```python
from build123d import *

# Parameters (mm, degrees)
SKETCH2_R           = 8.25
BOSS_EXTRUDE1_DEPTH = 5


with BuildPart() as part:
    # Sketch2 → Boss-Extrude1 (new, symmetric)
    with BuildSketch(Plane.XY.offset(-25)):
        Polygon((227.33813101, -85), (237.93813101, -85), (237.93813101, -64.7), (267.93813101, -64.7), (267.93813101, -144.7), (247.93813101, -164.7), (217.33813101, -164.7), (197.33813101, -144.7), (197.33813101, -64.7), (227.33813101, -64.7), align=None)
        with Locations(Location((232.63813101, -149.7, 0), (0, 0, 180))):
            Circle(SKETCH2_R, mode=Mode.SUBTRACT)
    extrude(amount=BOSS_EXTRUDE1_DEPTH, both=True)


solid = part.part
```
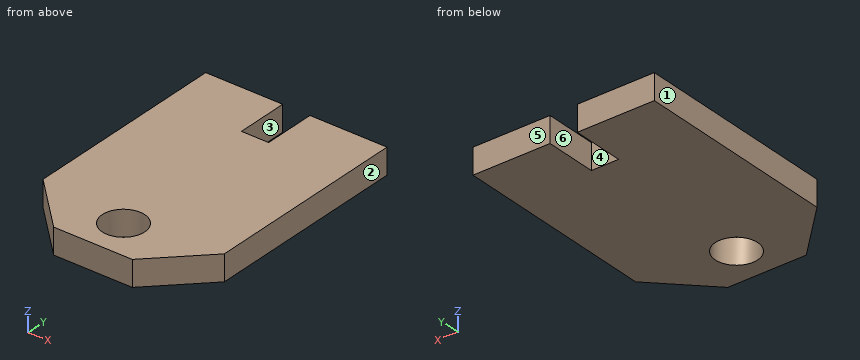
The model under review builds one solid part; all positions refer to its coordinate system, in mm. Face numbers are marked on the shaded views. A direction names the side the tool comes from. Round coordinates to 2 decimals unless told otherwise and drop trailing zeros. Loops run counter-clockwise (first coordinate to the right, second up) from the corner with the lowest first, then second, coordinate; pieces in that order, holes last. Notation, with made-up numbers: M 18.5,-19 L 66.5,-19 A23 ccw 66.5,13 Z; hole C 70.25,-2.75 d3. An arc over 180 degrees is marked long. Write item = value, one per line.
Item 1: The part is to be moulded in two halves that separate along X. For the marked faces 1, 2, 3 and 4, say which applies: released by +X, released by -X, zero draft, split by the parting line, or undercut.
Return value:
face_1 = released by -X
face_2 = released by +X
face_3 = undercut
face_4 = undercut
Item 2: Insertion check: P1, Ø15, axis at x = 232.64, y = -149.7, coming from the +Z side; P2, Ø3, axis at x = 231, z = -22.5, coming from the +Y side. Each pin has a flat end and moves straight along its axis. Give the tip position at first contact, or say it passes through.
Return value:
P1 = through
P2 = -85
Item 3: Take a section at A-A on z = -24.25. Write out the cut boundary in (x, y), then the cut area to 3 significant figures.
Return value:
outline = M 197.34,-144.7 L 217.34,-164.7 L 247.94,-164.7 L 267.94,-144.7 L 267.94,-64.7 L 237.94,-64.7 L 237.94,-85 L 227.34,-85 L 227.34,-64.7 L 197.34,-64.7 Z; hole C 232.64,-149.7 d16.5
area = 6,230 mm2
Item 4: Machinability: for the marked faces 5 and 6, which of the approach directions +Z, -Z, +X, -X, +Y, -Y give a long, thin tool a straight path to every point of the face, cutting with its end or side? Answer none if there is none.
Return value:
face_5 = +Z, -Z, +X, -X, +Y
face_6 = +Z, -Z, +Y
Item 5: Take a section at C-C on x = 236.5. Write out the cut boundary in (y, z).
Return value:
outline = M -164.7,-30 L -156.99,-30 L -156.99,-20 L -164.7,-20 Z; M -142.41,-30 L -85,-30 L -85,-20 L -142.41,-20 Z
Item 6: Take a section at D-D on x = 208.5. Write out the cut boundary in (y, z), then the cut area to 3 significant figures.
Return value:
outline = M -155.86,-30 L -64.7,-30 L -64.7,-20 L -155.86,-20 Z
area = 912 mm2
Item 7: Take a section at B-B on y = -149.7. Write out the cut boundary in (x, z), then the cut area to 3 significant figures.
Return value:
outline = M 202.34,-30 L 224.39,-30 L 224.39,-20 L 202.34,-20 Z; M 240.89,-30 L 262.94,-30 L 262.94,-20 L 240.89,-20 Z
area = 441 mm2
Item 8: For line 1 (X direction, y = -70, z = -23.75); line 2 (Y direction, x = 229, z = -23); line 3 (X direction, y = -149.7, z = -27.75), list the stretches that pass through material, from the lowest coordinate up. Write a range as [from, to].
Return value:
line_1 = [197.34, 227.34], [237.94, 267.94]
line_2 = [-164.7, -157.1], [-142.3, -85]
line_3 = [202.34, 224.39], [240.89, 262.94]
